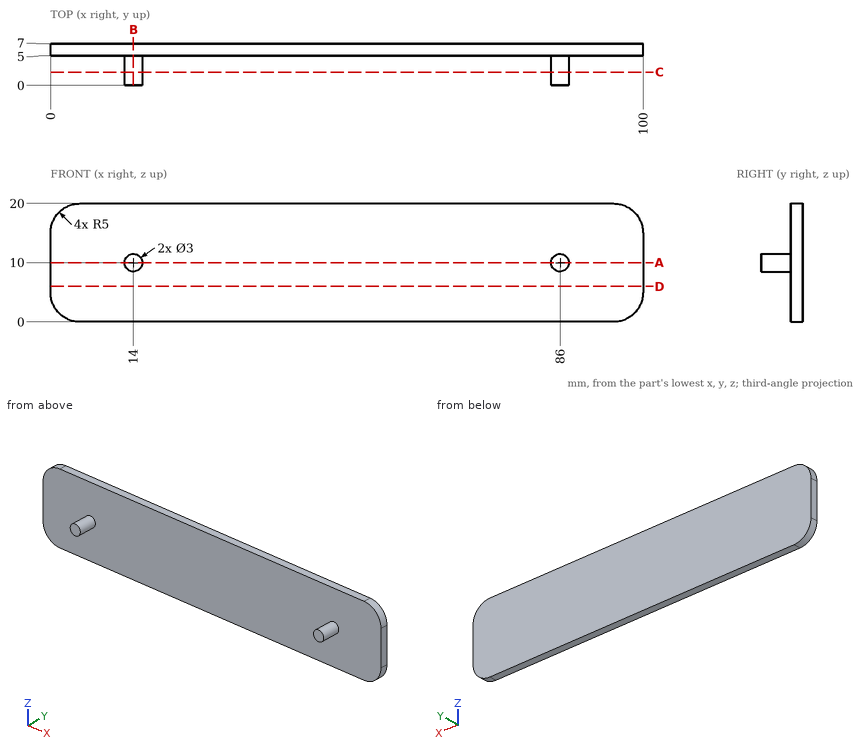
Check sheet for the drawn part. Datum: minimum x, y, z corner. Units: mm. Give positions to 0.01 mm unless a question says otherwise; leave off trailing zeros. Order: outer loops, then holes, each group sorted by start corner. A loop starts at its lowest first (then second) coordinate and runs counter-clockwise, first axis right, second up. Notation, with made-up numbers: (-31.5, 22.5) -> (-3.5, 22.5) arc R10 ccw to (-3.5, 41.5) -> close; hole circle Ø11 at (47, -1). An arc over 180 degrees is marked (long way). One line per item, written item: value.
(1) Sectioned sample at A-A on z = 10. Record the cut outline in (x, y).
Final values:
outline: (0, 5) -> (12.5, 5) -> (12.5, 0) -> (15.5, 0) -> (15.5, 5) -> (84.5, 5) -> (84.5, 0) -> (87.5, 0) -> (87.5, 5) -> (100, 5) -> (100, 7) -> (0, 7) -> close
(2) Sectioned sample at C-C on y = 2.25. Record the cut outline in (x, z).
Final values:
outline: circle Ø3 at (14, 10); circle Ø3 at (86, 10)
(3) Sectioned sample at D-D on z = 6. Record the cut outline in (x, y).
Final values:
outline: (0, 5) -> (100, 5) -> (100, 7) -> (0, 7) -> close
(4) Sectioned sample at B-B on x = 14. Record the cut outline in (y, z), then the cut area to 3 significant figures.
Final values:
outline: (0, 8.5) -> (5, 8.5) -> (5, 0) -> (7, 0) -> (7, 20) -> (5, 20) -> (5, 11.5) -> (0, 11.5) -> close
area: 55.0 mm^2
(5) Gauge pin test, flat ends, axial feed: pin 1 (10 mm diameter, centred on x = 66, z = 6.5, fed in from -Y); pin 2 (10 mm diameter, centred on x = 84.5, z = 7, fed in from -Y). Record the tip position at first contact, or that the pin passes through.
Final values:
pin 1: y = 5
pin 2: y = 0
(6) Scan lines: line 1 along X through (y, z) = (6.25, 4.75); line 2 along Y through (x, z) = (38.5, 9.5); line 3 along X through (y, z) = (5.75, 17.5). Record each from-to range of solid material in increasing order. Write a range as [from, to].
Final values:
line 1: [0.01, 99.99]
line 2: [5, 7]
line 3: [0.67, 99.33]
